```python
from build123d import *

# Parameters (mm, degrees)
EXTRUDE_1_DEPTH             = 15
HOLE_WIZARD_M121_D          = 10.2
HOLE_WIZARD_M121_DEPTH      = 15
HOLE_WIZARD_M81_D           = 6.8
HOLE_WIZARD_M81_DEPTH       = 15
HOLE_WIZARD_8_2_8_2_1_D     = 8.2
HOLE_WIZARD_8_2_8_2_1_DEPTH = 15
SKETCH_9_W                  = 8
SKETCH_9_H                  = 8
SKETCH_9_H_2                = 4
SKETCH_9_W_2                = 4
EXTRUDE_2_DEPTH             = 2
FILLET_1_R                  = 2


with BuildPart() as part:
    # Эскиз1 → Бобышка-Вытянуть1 (new body)
    with BuildSketch(Plane(origin=(0, 0, 0), x_dir=(1, 0, 0), z_dir=(0, 1, 0))):
        Polygon((0, 0), (0, 120), (40, 120), (120, 40), (120, 0), align=None)
    extrude(amount=EXTRUDE_1_DEPTH)

    # Отверстие обработанное метчиком M121
    with Locations(Plane(origin=(0, 15, 0), x_dir=(1, 0, 0), z_dir=(0, 1, 0))):
        with Locations((60, 60)):
            Hole(HOLE_WIZARD_M121_D / 2, depth=HOLE_WIZARD_M121_DEPTH)

    # Отверстие обработанное метчиком M81
    with Locations(Plane(origin=(0, 15, 0), x_dir=(1, 0, 0), z_dir=(0, 1, 0))):
        with Locations((50.454058454, 101.365746699), (101.365746699, 50.454058454), (69.545941546, 18.634253301), (18.634253301, 69.545941546)):
            Hole(HOLE_WIZARD_M81_D / 2, depth=HOLE_WIZARD_M81_DEPTH)

    # Диаметр отверстия Ø8.2 (8.2)1
    with Locations(Plane(origin=(0, 15, 0), x_dir=(1, 0, 0), z_dir=(0, 1, 0))):
        with Locations((20, 100), (20, 50), (20, 20), (50, 20), (100, 20)):
            Hole(HOLE_WIZARD_8_2_8_2_1_D / 2, depth=HOLE_WIZARD_8_2_8_2_1_DEPTH)

    # Эскиз9 → Бобышка-Вытянуть2 (add)
    with BuildSketch(Plane(origin=(0, 15, 0), x_dir=(1, 0, 0), z_dir=(0, 1, 0))):
        with Locations((20, 112)):
            Rectangle(SKETCH_9_W, SKETCH_9_H)
        with Locations((20, 81.545941546)):
            Rectangle(SKETCH_9_W, SKETCH_9_H)
        with Locations((20, 38)):
            Rectangle(SKETCH_9_W, SKETCH_9_H_2)
        with Locations((38, 20)):
            Rectangle(SKETCH_9_W_2, SKETCH_9_H)
        with Locations((81.545941546, 20)):
            Rectangle(SKETCH_9_W, SKETCH_9_H)
        with Locations((112, 20)):
            Rectangle(SKETCH_9_W, SKETCH_9_H)
    extrude(amount=EXTRUDE_2_DEPTH)

    # Скругление1
    fillet_1_edges = [part.edges().sort_by_distance(p)[0] for p in [
        (0, 7.5, 0),
        (0, 7.5, -120),
        (40, 7.5, -120),
        (120, 7.5, -40),
        (120, 7.5, 0),
    ]]
    fillet(fillet_1_edges, radius=FILLET_1_R)


solid = part.part
```
Verification items for the finished model (mm, model axes). Coordinates: 2 decimals unless noted, no trailing zeros. Loops run counter-clockwise (first coordinate to the right, second up) from the corner with the lowest first, then second, coordinate; pieces in that order, holes last. Notation, with made-up numbers: (-32.75, 43) - (9.25, 43) arc R17 cw to (9.25, 64) - close; hole circle Ø10 at (60.5, 86). An arc over 180 degrees is marked (long way). Put each result on its own line as item: value.
Item 1: Section check B-B (x = 60). Enter the section's corners in (y, z).
Conclusion:
outline: (0, -100) - (15, -100) - (15, -65.1) - (0, -65.1) - close; (0, -54.9) - (15, -54.9) - (15, 0) - (0, 0) - close
Item 2: Scan lines: line 1 along X through (y, z) = (11, -20); line 2 along X through (y, z) = (4, -102); line 3 along Z through (x, y) = (51, 11.75). Record each from-to range of solid material in increasing order.
Conclusion:
line 1: x = 0 to 15.9, 24.1 to 45.9, 54.1 to 66.43, 72.66 to 95.9, 104.1 to 120
line 2: x = 0 to 16.42, 23.58 to 47.11, 53.79 to 58
line 3: z = -109 to -104.72, -98.01 to -23.98, -16.02 to 0
Item 3: Section check A-A (z = -60). Enter the section's corners in (x, y).
Conclusion:
outline: (0, 0) - (54.9, 0) - (54.9, 15) - (0, 15) - close; (65.1, 0) - (100, 0) - (100, 15) - (65.1, 15) - close
Item 4: Draft check along X on faces 1 (the face through (48, 0, -48)), 2 (the face through (0, 7, -59)), 3 (the face through (50.9, 7.4, -16)). Enter one of: pulls with the +X half, pulls with the -X half, needs draft (parallel to the pull), parting line crosses it, or undercut.
Conclusion:
face 1: needs draft
face 2: pulls with the -X half
face 3: undercut
Item 5: Section check D-D (x = 100). Enter the section's corners in (y, z).
Conclusion:
outline: (0, -60) - (15, -60) - (15, -53.57) - (0, -53.57) - close; (0, -47.34) - (15, -47.34) - (15, -24.1) - (0, -24.1) - close; (0, -15.9) - (15, -15.9) - (15, 0) - (0, 0) - close
Item 6: Section check C-C (z = -100). Enter the section's corners in (x, y).
Conclusion:
outline: (0, 0) - (15.9, 0) - (15.9, 15) - (0, 15) - close; (24.1, 0) - (47.34, 0) - (47.34, 15) - (24.1, 15) - close; (53.57, 0) - (60, 0) - (60, 15) - (53.57, 15) - close
Item 7: Gauge pin test, flat ends, axial feed: pin 1 Ø2 at (y, z) = (4.5, -77) entering from +X; pin 2 Ø1.5 at (x, z) = (17, -31) entering from -Y; pin 3 Ø0.6 at (y, z) = (16.5, -37.5) entering from +X; pin 4 Ø5.5 at (x, z) = (50.45, -101.37) entering from +Y. Record the tip position at first contact, or that the pin passes through.
Conclusion:
pin 1: stops at x = 84
pin 2: stops at y = 0
pin 3: stops at x = 24
pin 4: passes through
